```python
from build123d import *

# Parameters (mm, degrees)
F0_R     = 40.327916
F0_R_2   = 21.082
F1_DEPTH = 44.45
F2_SIZE  = 2.54
F3_SIZE  = 5.08
F4_R     = 69.994365
F5_DEPTH = 44.451


with BuildPart() as f1:
    # F0 (on Front) → F1 (new body)
    with BuildSketch(Plane.XZ):
        Circle(F0_R)
        Circle(F0_R_2, mode=Mode.SUBTRACT)
    extrude(amount=F1_DEPTH)

    # F2
    f2_edges = [f1.edges().sort_by_distance(p)[0] for p in [
        (21.082, -22.225, 0),
        (-21.082, 0, 0),
        (-21.082, -44.45, 0),
    ]]
    chamfer(f2_edges, length=F2_SIZE)

    # F3
    f3_edges = [f1.edges().sort_by_distance(p)[0] for p in [
        (40.327916, -22.225, 0),
        (-40.327916, 0, 0),
        (-40.327916, -44.45, 0),
    ]]
    chamfer(f3_edges, length=F3_SIZE)

    # F4 (on Front) → F5 (cut, through all)
    with BuildSketch(Plane.XZ):
        Circle(F4_R)
        Polygon((28.276404, 28.815554), (39.093203, -10.080307), (10.8168, -38.895861), (-28.276404, -28.815554), (-39.093203, 10.080307), (-10.8168, 38.895861), align=None, mode=Mode.SUBTRACT)
    extrude(amount=F5_DEPTH, mode=Mode.SUBTRACT)


solid = f1.part
```
Check sheet for the modelled part. Datum: model origin and axes. Units: mm. Round coordinates to 2 decimals unless told otherwise and drop trailing zeros. Write each loop counter-clockwise with the first axis right and the second up, starting at its lowest first coordinate (ties: lowest second). Pieces come first, ordered by that corner, then holes. Notation, with made-up numbers: M -6.5,-28 L 17.5,-28 A30 ccw 17.5,-3 Z; hole C 40.25,-12.75 d2. An arc over 180 degrees is marked long. Write item = value, one per line. Start each with the question number.
1. Section check C-C, the plane x = 0. Record the cut outline in (y, z), then the cut area to 3 significant figures.
2. Scan lines: line 1 (X direction, y = -30.5, z = 16); line 2 (Z direction, x = 0, y = -31.5); line 3 (Z direction, x = 18, y = -32) (3 decimals). Record each from-to range of solid material in increasing order. Write a range as [from, to].
3. Section check A-A, the plane y = -28.5. Record the cut outline in (x, z).
4. Section check B-B, the plane z = 0. Record the cut outline in (x, y), then the cut area to 3 significant figures.
5. Section check D-D, the plane y = -3.5. Record the cut outline in (x, z), then the cut area to 3 significant figures.
6. Release check for a two-part mould opening along X. For faces 1 (the conical face through (11.4, -2.4, 17.9)), 2 (the flat face through (33.61, -21.91, 9.64)), 3 (the flat face through (-8.457, -21.914, -33.926)) record: pulls with the +X half, pulls with the -X half, needs draft (parallel to the pull), parting line crosses it, or undercut.
7. Gauge pin test, flat ends, axial feed: pin 1 (3 mm diameter, centred on x = -15.5, y = -37, fed in from -Z); pin 2 (4 mm diameter, centred on x = 15, y = -36, fed in from +Z); pin 3 (1.5 mm diameter, centred on x = -13, y = -35, fed in from +Z). Record the tip position at first contact, or that the pin passes through.
Results found:
q1.outline = M -44.45,-35.25 L -43.59,-36.11 L -0.86,-36.11 L 0,-35.25 L 0,-23.62 L -2.54,-21.08 L -41.91,-21.08 L -44.45,-23.62 Z; M -44.45,23.62 L -41.91,21.08 L -2.54,21.08 L 0,23.62 L 0,35.25 L -0.86,36.11 L -43.59,36.11 L -44.45,35.25 Z
q1.area = 1,320 mm^2
q2.line_1 = [-33.28, -13.73], [13.73, 31.84]
q2.line_2 = [-36.11, -21.08], [21.08, 36.11]
q2.line_3 = [-31.576, -10.975], [10.975, 31.465]
q3.outline = M -39.07,10 L -28.3,-28.73 A40.33 ccw -28.19,-28.84 L 10.73,-38.87 A40.33 ccw 10.88,-38.83 L 39.03,-10.14 A40.33 ccw 39.07,-10 L 28.3,28.73 A40.33 ccw 28.19,28.84 L -10.73,38.87 A40.33 ccw -10.88,38.83 L -39.03,10.14 A40.33 ccw Z; hole C 0,0 d42.16
q4.outline = M -36.29,-43.41 L -35.25,-44.45 L -23.62,-44.45 L -21.08,-41.91 L -21.08,-2.54 L -23.62,0 L -35.25,0 L -36.29,-1.04 Z; M 21.08,-41.91 L 23.62,-44.45 L 35.25,-44.45 L 36.29,-43.41 L 36.29,-1.04 L 35.25,0 L 23.62,0 L 21.08,-2.54 Z
q4.area = 1,340 mm^2
q5.outline = M -38.16,6.72 L -29.21,-25.46 A38.75 ccw -24.9,-29.69 L 7.44,-38.03 A38.75 ccw 13.26,-36.41 L 36.65,-12.57 A38.75 ccw 38.16,-6.72 L 29.21,25.46 A38.75 ccw 24.9,29.69 L -7.44,38.03 A38.75 ccw -13.26,36.41 L -36.65,12.57 A38.75 ccw Z; hole C 0,0 d42.16
q5.area = 2,810 mm^2
q6.face_1 = undercut
q6.face_2 = pulls with the +X half
q6.face_3 = pulls with the -X half
q7.pin_1 = -32.5
q7.pin_2 = 32.75
q7.pin_3 = 37.44
